```python
from build123d import *

# Parameters (mm, degrees)
EXTRUDE_1_DEPTH     = 47
SKETCH_2_R          = 4
CUT_EXTRUDE_1_DEPTH = 10


with BuildPart() as part:
    # Эскиз1 → Вытянуть-Тонкостенный1 (new body)
    with BuildSketch(Plane(origin=(0, 0, 0), x_dir=(0, 0, -1), z_dir=(1, 0, 0))):
        Polygon((-40.5, 0), (-20.5, 0), (-20.5, 10.25), (20.5, 10.25), (20.5, 0), (40.5, 0), (40.5, 2), (22.5, 2), (22.5, 12.25), (-22.5, 12.25), (-22.5, 2), (-40.5, 2), align=None)
    extrude(amount=EXTRUDE_1_DEPTH)

    # Эскиз2 → Вырез-Вытянуть1 (cut)
    with BuildSketch(Plane.XZ):
        with Locations((10, 30)):
            Circle(SKETCH_2_R)
        with Locations((30, 30)):
            Circle(SKETCH_2_R)
        with Locations((30, -30)):
            Circle(SKETCH_2_R)
        with Locations((10, -30)):
            Circle(SKETCH_2_R)
    extrude(amount=-CUT_EXTRUDE_1_DEPTH, mode=Mode.SUBTRACT)


solid = part.part
```
Verification items for the finished model (mm, model axes). A direction names the side the tool comes from. Give positions to 0.01 mm unless a question says otherwise; leave off trailing zeros. Loops run counter-clockwise (first coordinate to the right, second up) from the corner with the lowest first, then second, coordinate; pieces in that order, holes last. Notation, with made-up numbers: M 73.5,-30 L 88.5,-30 A24 cw 88.5,3 Z; hole C 6.5,-37.5 d10. An arc over 180 degrees is marked long. Return JSON: item names as keys, results as strings.
1) Section check B-B, the plane x = 10. Enter the section's corners in (y, z).
Findings:
{"outline": "M 0,-40.5 L 2,-40.5 L 2,-34 L 0,-34 Z; M 0,-26 L 2,-26 L 2,-22.5 L 12.25,-22.5 L 12.25,22.5 L 2,22.5 L 2,26 L 0,26 L 0,20.5 L 10.25,20.5 L 10.25,-20.5 L 0,-20.5 Z; M 0,34 L 2,34 L 2,40.5 L 0,40.5 Z"}
2) Material ranges on L1, parallel to Z at x = 30, y = 1.1; L2, parallel to Z at x = 39.5, y = 6.75; L3, parallel to Z at x = 20.5, y = 1, recorded low to high. Write a range as [from, to].
Findings:
{"L1": "z = [-40.5, -34], [-26, -20.5], [20.5, 26], [34, 40.5]", "L2": "z = [-22.5, -20.5], [20.5, 22.5]", "L3": "z = [-40.5, -20.5], [20.5, 40.5]"}
3) Section check D-D, the plane y = 1. Enter the section's corners in (x, z).
Findings:
{"outline": "M 0,-40.5 L 47,-40.5 L 47,-20.5 L 0,-20.5 Z; M 0,20.5 L 47,20.5 L 47,40.5 L 0,40.5 Z; hole C 10,-30 d8; hole C 10,30 d8; hole C 30,-30 d8; hole C 30,30 d8"}
4) Gauge pin test, flat ends, axial feed: P1, Ø9, axis at x = 35, z = -33, coming from the +Y side; P2, Ø4, axis at x = 37, y = 7.5, coming from the +Z side; P3, Ø6, axis at y = 4.5, z = -9, coming from the +X side; P4, Ø1.5, axis at x = 15.5, y = 6.5, coming from the -Z side. Record the tip position at first contact, or that the pin passes through.
Findings:
{"P1": "stops at y = 2", "P2": "stops at z = 22.5", "P3": "passes through", "P4": "stops at z = -22.5"}
5) Mould release check, pull along Z, two halves, no side actions. Record for faces 1 (the flat face through (23, 7, 22.5)), 2 (the flat face through (23, 0, 31)), 3 (the cylindrical face through (9.479, 0.986, 33.966)): released by +Z, released by -Z, zero draft, split by the parting line, or undercut.
Findings:
{"face 1": "released by +Z", "face 2": "zero draft", "face 3": "undercut"}
6) Tool access check on faces 4 (the flat face through (0, 11, 0)), 5 (the flat face through (23, 5, 20.5)), 6 (the flat face through (23, 2, 31)), 7 (the cylindrical face through (9.479, 0.986, -26.034)), 8 (the flat face through (23, 7, -22.5)). Record the directions out of +Z, -Z, +X, -X, +Y, -Y that give a thin tool (end or side, any length) a straight path to the whole face; none if there is none.
Findings:
{"face 4": "+Z, -Z, -X, +Y, -Y", "face 5": "+X, -X, -Y", "face 6": "+Z, +X, -X, +Y", "face 7": "+Y, -Y", "face 8": "-Z, +X, -X, +Y"}
7) Section check A-A, the plane z = 30. Enter the section's corners in (x, y).
Findings:
{"outline": "M 0,0 L 6,0 L 6,2 L 0,2 Z; M 14,0 L 26,0 L 26,2 L 14,2 Z; M 34,0 L 47,0 L 47,2 L 34,2 Z"}
8) Section check C-C, the plane y = 5. Enter the section's corners in (x, z).
Findings:
{"outline": "M 0,-22.5 L 47,-22.5 L 47,-20.5 L 0,-20.5 Z; M 0,20.5 L 47,20.5 L 47,22.5 L 0,22.5 Z"}
